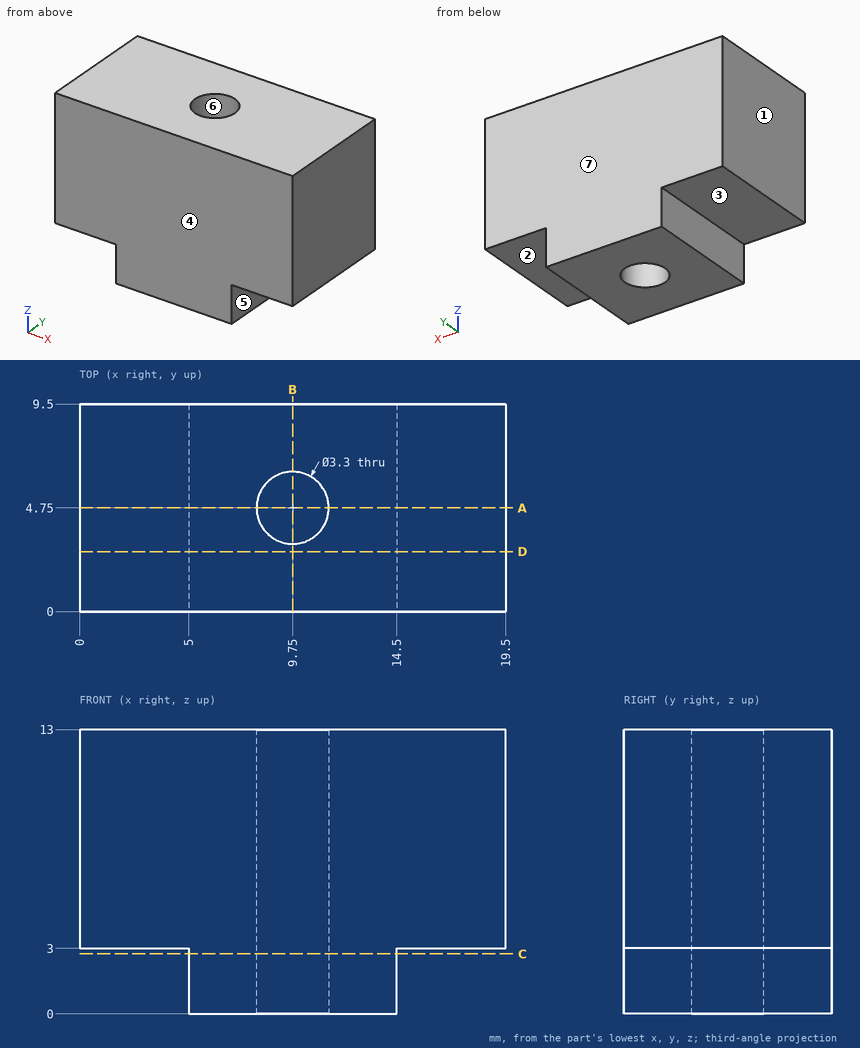
Here's the drawing with two shaded views (mm, measured from the low corner). I have some questions. A direction names the side the tool comes from. Coordinates: 2 decimals unless noted, no trailing zeros. Loops run counter-clockwise (first coordinate to the right, second up) from the corner with the lowest first, then second, coordinate; pieces in that order, holes last.
Item 1: Suppose I cut it at B-B (x = 9.75). Please give me the cut outline in (y, z), then the cut area to 3 significant figures.
Answers below:
outline: (0, 0) - (3.1, 0) - (3.1, 13) - (0, 13) - close; (6.4, 0) - (9.5, 0) - (9.5, 13) - (6.4, 13) - close
area: 80.6 mm2
Item 2: Suppose I cut it at D-D (y = 2.75). Please give me the cut outline in (x, z).
Answers below:
outline: (0, 3) - (5, 3) - (5, 0) - (14.5, 0) - (14.5, 3) - (19.5, 3) - (19.5, 13) - (0, 13) - close
Item 3: Suppose I cut it at C-C (z = 2.75). Please give me the cut outline in (x, y), then the cut area to 3 significant figures.
Answers below:
outline: (5, 0) - (14.5, 0) - (14.5, 9.5) - (5, 9.5) - close; hole circle Ø3.3 at (9.75, 4.75)
area: 81.7 mm2
Item 4: Please list where these lines run through material, in increasing order: L1, parallel to Y at x = 9.75, z = 9; L2, parallel to Y at x = 10.25, z = 1.5; L3, parallel to Z at x = 18.5, y = 4.75.
Answers below:
L1: y = 0 to 3.1, 6.4 to 9.5
L2: y = 0 to 3.18, 6.32 to 9.5
L3: z = 3 to 13
Item 5: Suppose I cut it at A-A (y = 4.75). Please give me the cut outline in (x, z), then the cut area to 3 significant figures.
Answers below:
outline: (0, 3) - (5, 3) - (5, 0) - (8.1, 0) - (8.1, 13) - (0, 13) - close; (11.4, 0) - (14.5, 0) - (14.5, 3) - (19.5, 3) - (19.5, 13) - (11.4, 13) - close
area: 181 mm2
Item 6: Which directions (+Z, -Z, +X, -X, +Y, -Y) give clear straight access to the entire face, cutting with the end or side of a thin tool? Please do the marked faces 1, 2 and 3.
Answers below:
face 1: +Z, -Z, -X, +Y, -Y
face 2: -Z, +X, +Y, -Y
face 3: -Z, -X, +Y, -Y
Item 7: I'm going to push flat-ended pins straight in: pin 1 (1.5 mm diameter, centred on y = 4.5, z = 2, fed in from +X); pin 2 (4 mm diameter, centred on x = 2, y = 7, fed in from -Z); pin 3 (2.5 mm diameter, centred on y = 6.5, z = 1, fed in from -X). Where does each tip first touch, or does it pass through?
Answers below:
pin 1: stops at x = 14.5
pin 2: stops at z = 3
pin 3: stops at x = 5
Item 8: If we mould it in two halves opening along Y, with no side actions, what happens to the marked faces 4, 5, 6 and 7? For each: released by +Y, released by -Y, zero draft, split by the parting line, or undercut.
Answers below:
face 4: released by -Y
face 5: zero draft
face 6: undercut
face 7: released by +Y
